Verification items for the finished model (mm, model axes). A direction names the side the tool comes from. Give positions to 0.01 mm unless a question says otherwise; leave off trailing zeros. Write each loop counter-clockwise with the first axis right and the second up, starting at its lowest first coordinate (ties: lowest second). Pieces come first, ordered by that corner, then holes. Notation, with made-up numbers: (3, -5.75) - (41, -5.75) arc R16 ccw to (41, 14.25) - close; hole circle Ø5 at (74, 80). An arc over 180 degrees is marked (long way). Answer as a JSON object with one key per item and string values. Group by question number.
Item 1: Sectioned sample at C-C, the plane z = 5.2. Record the boundary of the cut face in (x, y).
Item 2: Sectioned sample at A-A, the plane y = 2.5. Record the boundary of the cut face in (x, z).
Item 3: Sectioned sample at B-B, the plane x = 2. Record the boundary of the cut face in (y, z), and give its area (3 significant figures).
Item 4: Tool access check on faces 5 (the face through (4, 3, 0)), 6 (the face through (4.8, 2, 4)). Record the directions out of +Z, -Z, +X, -X, +Y, -Y that give a thin tool (end or side, any length) a straight path to the whole face; none if there is none.
Item 5: Scan lines: line 1 along Y through (x, z) = (5.15, 5.2); line 2 along X through (y, z) = (0.6, 2.5); line 3 along Z through (x, y) = (3.2, 3.5). Record each from-to range of solid material in increasing order. Write a range as [from, to].
Item 6: Draft check along Y on faces 1 (the face through (0, 3, 1)), 2 (the face through (1.263, 3.176, 0.592)), 3 (the face through (5.392, 2.117, 6.124)), 4 (the face through (5, 5, 2)). Enter one of: +Y half, -Y half, draft (parallel to the pull), parting line (faces both ways), or undercut.
Item 7: Sectioned sample at D-D, the plane z = 1. Record the boundary of the cut face in (x, y), and give its area (3 significant figures).
Item 8: Go/stop test with flat-tipped pins: pin 1 (2 mm diameter, centred on y = 3.5, z = 4.5, fed in from -X); pin 2 (1 mm diameter, centred on x = 2, y = 0.5, fed in from +Z). Record where each tip stops, or that it passes through.
```python
from build123d import *

# Parameters (mm, degrees)
SKETCH_1_R          = 1
EXTRUDE_1_DEPTH     = 1.2
SKETCH_2_W          = 1.2
SKETCH_2_H          = 5
EXTRUDE_2_DEPTH     = 6
FILLET_1_R          = 1
SKETCH_4_R          = 1
CUT_EXTRUDE_1_DEPTH = 2


with BuildPart() as part:
    # 草图1 → 凸台-拉伸1 (new body)
    with BuildSketch(Plane.XY):
        with BuildLine():
            Line((1, 0), (6, 0))
            Line((6, 0), (6, 5))
            Line((6, 5), (1, 5))
            ThreePointArc((1, 5), (0.292893219, 4.707106781), (0, 4))
            Line((0, 4), (0, 1))
            ThreePointArc((0, 1), (0.292893219, 0.292893219), (1, 0))
        make_face()
        with Locations((2, 2.5)):
            Circle(SKETCH_1_R, mode=Mode.SUBTRACT)
    extrude(amount=EXTRUDE_1_DEPTH)

    # 草图2 → 凸台-拉伸2 (add)
    with BuildSketch(Plane(origin=(0, 0, 1.2), x_dir=(-1, 0, 0), z_dir=(0, 0, -1))):
        with Locations((-5.4, 2.5)):
            Rectangle(SKETCH_2_W, SKETCH_2_H)
    extrude(amount=-EXTRUDE_2_DEPTH)

    # 圆角1
    fillet_1_edges = [part.edges().sort_by_distance(p)[0] for p in [
        (5.4, 0, 7.2),
        (5.4, 5, 7.2),
    ]]
    fillet(fillet_1_edges, radius=FILLET_1_R)

    # 草图4 → 切除-拉伸1 (cut)
    with BuildSketch(Plane.ZY.offset(-4.8)):
        with Locations((5.2, 2.5)):
            Circle(SKETCH_4_R)
    extrude(amount=-CUT_EXTRUDE_1_DEPTH, mode=Mode.SUBTRACT)


solid = part.part
```
Geometry check:
{
 "1": {"outline": "(4.8, 0) - (6, 0) - (6, 1.5) - (4.8, 1.5) - close; (4.8, 3.5) - (6, 3.5) - (6, 5) - (4.8, 5) - close"},
 "2": {"outline": "(0, 0) - (1, 0) - (1, 1.2) - (0, 1.2) - close; (3, 0) - (6, 0) - (6, 4.2) - (4.8, 4.2) - (4.8, 1.2) - (3, 1.2) - close; (4.8, 6.2) - (6, 6.2) - (6, 7.2) - (4.8, 7.2) - close"},
 "3": {"outline": "(0, 0) - (1.5, 0) - (1.5, 1.2) - (0, 1.2) - close; (3.5, 0) - (5, 0) - (5, 1.2) - (3.5, 1.2) - close", "area": "3.60 mm^2"},
 "4": {"face 5": "-Z, +X, -X, +Y, -Y", "face 6": "+Z, -X, +Y, -Y"},
 "5": {"line 1": "[0, 1.5], [3.5, 5]", "line 2": "[4.8, 6]", "line 3": "[0, 1.2]"},
 "6": {"face 1": "draft", "face 2": "undercut", "face 3": "undercut", "face 4": "+Y half"},
 "7": {"outline": "(0, 1) arc R1 ccw to (1, 0) - (6, 0) - (6, 5) - (1, 5) arc R1 ccw to (0, 4) - close; hole circle Ø2 at (2, 2.5)", "area": "26.4 mm^2"},
 "8": {"pin 1": "x = 4.8", "pin 2": "z = 1.2"}
}
